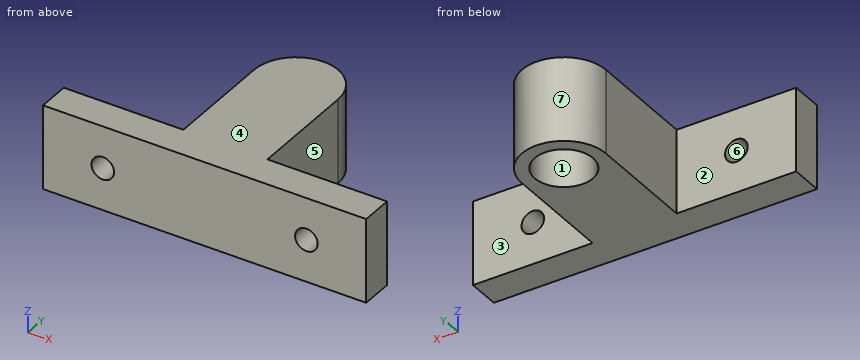
Autodesk Inventor part; units mm, degrees
ref_plane "Work Plane1" through (-2, -2, 20) normal (0, 0, 1) x (1, 0, 0)
ref_plane "YZ Plane" through (0, 0, 0) normal (1, 0, 0) x (0, 1, 0)
ref_plane "XZ Plane" through (0, 0, 0) normal (0, 1, 0) x (-1, 0, 0)
sketch "Sketch1" plane through (0, 0, 0) normal (0, 0, 1) x (1, 0, 0)
  circle A0 centre (0, 11) radius 4 construction
  circle A1 centre (0, 11) radius 4.5
  line L0 (200.3677, 25.2343) -> (-185.7345, -79.2887) construction
  line L1 (200.3677, 25.2343) -> (210.1768, -11) construction
  line L2 (-204.2212, -11) -> (210.1768, -11) construction
  line L3 (-185.7345, -79.2887) -> (-204.2212, -11) construction
  arc A2 (6.5, 11) -> (-6.5, 11) centre (0, 11) ccw
  line L4 (6.5, 11) -> (6.5, -6)
  line L5 (-6.5, 11) -> (-6.5, -6)
  line L6 (25, -6) -> (25, -11)
  line L7 (-25, -6) -> (-25, -11)
  line L8 (-25, -11) -> (25, -11)
  line L9 (-25, -6) -> (-6.5, -6)
  line L10 (6.5, -6) -> (25, -6)
  point P0 (0, 0)
  dimension "d0" = 0.5
  dimension "d1" = 2
  dimension "d3" = 18.5
  dimension "d4" = 13
  dimension "d5" = 18.5
  dimension "d6" = 5
  dimension "d7" = 5
  dimension "d20" = 22
  dimension "d21" = 11
  dimension "d22" = 25
  dimension "d23" = 50
ref_plane "Work Plane1" through (-2, -2, 20) normal (0, 0, 1) x (1, 0, 0)
extrude "Tykkelse" add sketch "Sketch1" along normal blind 13
sketch "Sketch2" plane through (-25, -11, 0) normal (0, -1, 0) x (1, 0, 0)
  line L0 (0, 13) -> (50, 13)
  line L1 (0, 0) -> (0, 13)
  line L2 (18.5, 0) -> (0, 0)
  line L3 (0, 0) -> (0, 13)
  line L4 (18.5, 13) -> (0, 13)
  line L5 (18.5, 0) -> (18.5, 13)
  line L6 (50, 0) -> (31.5, 0)
  line L7 (31.5, 0) -> (31.5, 13)
  line L8 (50, 13) -> (31.5, 13)
  line L9 (50, 0) -> (50, 13)
  circle A0 centre (9.25, 6.5) radius 1.75
  circle A1 centre (40.75, 6.5) radius 1.75
  point P0 (25, 0)
  dimension "d10" = 3.5
  dimension "d11" = 3.5
  dimension "d12" = 9.25
  dimension "d13" = 9.25
  dimension "d14" = 6.5
  dimension "d15" = 6.5
  dimension "d16" = 9.25
  dimension "d17" = 6.5
extrude "Monteringshuller" cut sketch "Sketch2" against normal up to surface (5 mm away) contours A0 | A1
sketch "Sketch3" plane through (0, 0, 13) normal (0, 0, 1) x (1, 0, 0)
  circle A0 centre (0, 11) radius 4.5 construction
  arc A1 (6.5, 11) -> (-6.5, 11) centre (0, 11) ccw construction
  line L0 (-6.5, 11) -> (-6.5, -6) construction
  line L1 (-6.5, -6) -> (-25, -6) construction
  line L2 (-25, -6) -> (-25, -11) construction
  line L3 (-25, -11) -> (25, -11) construction
  line L4 (25, -11) -> (25, -6) construction
  line L5 (25, -6) -> (6.5, -6) construction
  line L6 (6.5, -6) -> (6.5, 11) construction
  circle A2 centre (0, 11) radius 4.5
  point P0 (0, 0)
extrude "Fyld hul" add sketch "Sketch3" against normal blind 2
equation "\"d5\" = d3"
equation "\"d7\" = d6"
equation "\"d11\" = d10"
equation "\"d12\" = d13"
equation "\"d14\" = d15"
equation "\"d16\" = d12"
equation "\"d17\" = d14"
properties part number "Z-Gevind-Holder" material "PC/ABS Plastic"
Build history of the part. All positions in model axes, mm. Face numbers are marked on the shaded views. A direction names the side the tool comes from. Give positions to 0.01 mm unless a question says otherwise; leave off trailing zeros. Order: outer loops, then holes, each group sorted by start corner. A loop starts at its lowest first (then second) coordinate and runs counter-clockwise, first axis right, second up. Notation, with made-up numbers: M 69,-23.5 L 113,-23.5 A29 cw 113,4.5 Z; hole C 87.25,-5 d7. An arc over 180 degrees is marked long. Write item = value, one per line. Start each with the question number.
(1) Slice it at C-C on z = 2. Write the cut outline in (x, y).
(2) Slice it at A-A on z = 6.5. Write the cut outline in (x, y).
(3) Slice it at D-D on x = -2.5. Write the cut outline in (y, z).
(4) Slice it at B-B on x = -15.75. Write the cut outline in (y, z), plus the area to 3 significant figures.
(5) Which spindle directions (+Z, -Z, +X, -X, +Y, -Y) get a long thin tool onto all of the face, cutting with end or side? Do the marked faces 1, 2 and 3. Say none if no direction does.
(6) Two-plate mould, pull along X, no slides. Class the marked faces 4, 5, 6 and 7: released by +X, released by -X, zero draft, split by the parting line, or undercut.
(7) Pin check, flat tips, straight feed: pin 1 Ø1.5 at (y, z) = (-3, 2.5) entering from +X; pin 2 Ø5.5 at (x, y) = (0, 11) entering from -Z; pin 3 Ø4 at (y, z) = (4, 9.5) entering from -X. Stop position of each tip, or through.
(8) Probe L1, parallel to Y at x = 0, z = 8.25; L2, parallel to Z at x = -15.75, y = -8.85; L3, parallel to Z at x = -2.5, y = 8. List the from-to ranges inside material, lowest first. Write a range as [from, to].
Responses:
q1.outline = M -25,-11 L 25,-11 L 25,-6 L 6.5,-6 L 6.5,11 A6.5 ccw -6.5,11 L -6.5,-6 L -25,-6 Z; hole C 0,11 d9
q2.outline = M -25,-11 L -17.5,-11 L -17.5,-6 L -25,-6 Z; M -14,-11 L 14,-11 L 14,-6 L 6.5,-6 L 6.5,11 A6.5 ccw -6.5,11 L -6.5,-6 L -14,-6 Z; M 17.5,-11 L 25,-11 L 25,-6 L 17.5,-6 Z; hole C 0,11 d9
q3.outline = M -11,0 L 7.26,0 L 7.26,11 L 14.74,11 L 14.74,0 L 17,0 L 17,13 L -11,13 Z
q4.outline = M -11,0 L -6,0 L -6,4.75 L -11,4.75 Z; M -11,8.25 L -6,8.25 L -6,13 L -11,13 Z
q4.area = 47.5 mm2
q5.face_1 = -Z
q5.face_2 = +Z, -Z, -X, +Y
q5.face_3 = +Z, -Z, +X, +Y
q6.face_4 = zero draft
q6.face_5 = released by +X
q6.face_6 = undercut
q6.face_7 = split by the parting line
q7.pin_1 = 6.5
q7.pin_2 = 11
q7.pin_3 = -6.5
q8.L1 = [-11, 6.5], [15.5, 17.5]
q8.L2 = [0, 4.75], [8.25, 13]
q8.L3 = [11, 13]
